Geometry check sheet. Reference: the model listing, model coordinates, mm. Face numbers are marked on the shaded views. Round coordinates to 2 decimals unless told otherwise and drop trailing zeros. Write each loop counter-clockwise with the first axis right and the second up, starting at its lowest first coordinate (ties: lowest second). Pieces come first, ordered by that corner, then holes. Notation, with made-up numbers: M -17.5,74 L 35.5,74 A21 ccw 35.5,92 Z; hole C 41,80.25 d11. An arc over 180 degrees is marked long. Use a Markdown table: item, result.
```python
from build123d import *

# Parameters (mm, degrees)
SKETCH1_W               = 22.5
SKETCH1_H               = 14
EXTRUDE1_DEPTH          = 7.2
SKETCH6_R               = 0.45
CUT_EXTRUDE1_DEPTH      = 0.1
CUT_EXTRUDE2_DEPTH      = 1
CUT_EXTRUDE2_DEPTH_BACK = 23.5
CUT_EXTRUDE3_DEPTH      = 1
CUT_EXTRUDE3_DEPTH_BACK = 15
LPATTERN1_COUNT         = 2
LPATTERN1_PITCH         = 7.5
LPATTERN2_COUNT         = 2
LPATTERN2_PITCH         = 7.5
BOSS_EXTRUDE4_START     = -1
SKETCH11_R              = 0.225
BOSS_EXTRUDE4_DEPTH     = 7.1
LPATTERN3_COUNT         = 6
LPATTERN3_PITCH         = 2.54
LPATTERN3_COUNT_DIR2    = 2
LPATTERN3_PITCH_DIR2    = 10.16


with BuildPart() as part:
    # Sketch1 → Extrude1 (new body)
    with BuildSketch(Plane(origin=(0, 0, 0), x_dir=(1, 0, 0), z_dir=(0, 1, 0))):
        Rectangle(SKETCH1_W, SKETCH1_H)
    extrude(amount=-EXTRUDE1_DEPTH)

    # Sketch6 → Cut-Extrude1 (cut)
    with BuildSketch(Plane(origin=(0, 0, 0), x_dir=(-1, 0, 0), z_dir=(0, 1, 0))):
        with Locations((-2.828914589, 5.1)):
            Circle(SKETCH6_R)
        Polygon((1.615140342, 0.645647316), (1.874984591, 3.615680666), (2.672057265, 4.346063205), (2.736318521, 4.281801948), (2.412096101, 0.575922722), (1.978755924, 0.212307139), align=None)
        Polygon((-2.08510989, 4.246446609), (-2.404999919, 0.590086851), (-2.118563171, 0.248724827), (-1.593244842, 0.689519243), (-1.335889658, 3.631102448), (-1.988382771, 4.343173729), align=None)
        Polygon((-2.751982586, -4.346963991), (-2.828914589, -4.255280001), (-2.499336567, -0.488185972), (-2.097293847, -0.150832074), (-1.707416581, -0.615469707), (-1.976986224, -3.696664829), align=None)
        Polygon((-2.591285684, -4.538475102), (-1.79792785, -3.872768836), (1.154576659, -3.872768836), (1.713170541, -4.538475102), (1.639848023, -4.6), (-2.539660165, -4.6), align=None)
        Polygon((1.560181456, -0.4), (1.954104558, -0.069459271), (1.560181456, 0.4), (-1.627135675, 0.4), (-2.021058776, 0.069459271), (-1.627135675, -0.4), align=None)
        Polygon((2.495112157, 4.523008313), (2.41812047, 4.6), (-1.7315565, 4.6), (-1.811437663, 4.520118836), (-1.151570324, 3.8), (1.706087039, 3.8), align=None)
        Polygon((1.982853172, -0.306417777), (2.30166085, -0.686357973), (1.984568022, -4.310745576), (1.904681652, -4.377778199), (1.244483112, -3.590984217), (1.496113015, -0.714841264), align=None)
    cut_extrude1 = extrude(amount=-CUT_EXTRUDE1_DEPTH, mode=Mode.SUBTRACT)

    # Sketch12 → Cut-Extrude2 (cut, two sides)
    with BuildSketch(Plane.ZY.offset(11.25)) as cut_extrude2_sk:
        Polygon((-20.043427491, -42.781711537), (-5.305, -7.2), (-4.890786438, -6.2), (4.890786438, -6.2), (5.305, -7.2), (20.043427491, -42.781711537), (20.043427491, -119.808445619), (-20.043427491, -119.808445619), align=None)
    extrude(amount=CUT_EXTRUDE2_DEPTH, mode=Mode.SUBTRACT)
    extrude(cut_extrude2_sk.sketch, amount=-CUT_EXTRUDE2_DEPTH_BACK, mode=Mode.SUBTRACT)

    # Sketch13 → Cut-Extrude3 (cut, two sides)
    with BuildSketch(Plane(origin=(0, 0, -7), x_dir=(-1, 0, 0), z_dir=(0, 0, -1))) as cut_extrude3_sk:
        Polygon((-32.290672921, -56.074755802), (-9.5, -7.2), (-9.033692342, -6.2), (9.033692342, -6.2), (9.5, -7.2), (32.290672921, -56.074755802), (32.290672921, -163.929408496), (-32.290672921, -163.929408496), align=None)
    extrude(amount=CUT_EXTRUDE3_DEPTH, mode=Mode.SUBTRACT)
    extrude(cut_extrude3_sk.sketch, amount=-CUT_EXTRUDE3_DEPTH_BACK, mode=Mode.SUBTRACT)

    # LPattern1: Cut-Extrude1 ×2
    with Locations(*[(i * LPATTERN1_PITCH, 0, 0) for i in range(1, LPATTERN1_COUNT)]):
        add(cut_extrude1, mode=Mode.SUBTRACT)

    # LPattern2: Cut-Extrude1 ×2
    with Locations(*[(-i * LPATTERN2_PITCH, 0, 0) for i in range(1, LPATTERN2_COUNT)]):
        add(cut_extrude1, mode=Mode.SUBTRACT)

    # Sketch11 → Boss-Extrude4 (add)
    with BuildSketch(Plane.XZ.offset(7.2).offset(BOSS_EXTRUDE4_START)):
        with Locations((6.35, 5.08)):
            Circle(SKETCH11_R)
    boss_extrude4 = extrude(amount=BOSS_EXTRUDE4_DEPTH)

    # LPattern3: Boss-Extrude4 6 × 2
    with Locations(*[(-i * LPATTERN3_PITCH, 0, -j * LPATTERN3_PITCH_DIR2) for i in range(LPATTERN3_COUNT) for j in range(LPATTERN3_COUNT_DIR2) if (i, j) != (0, 0)]):
        add(boss_extrude4)


solid = part.part
```
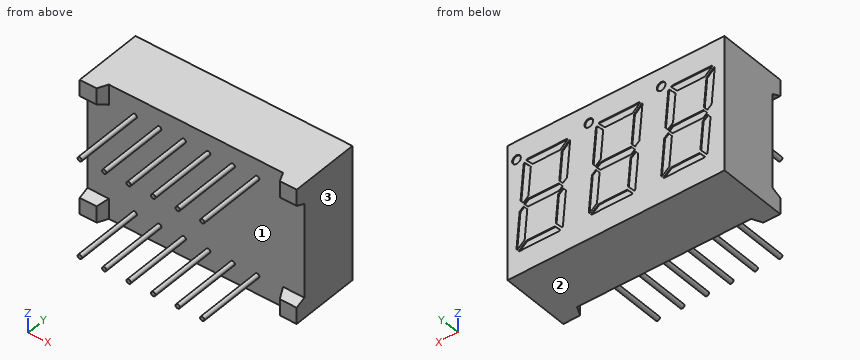
Item 1: Cross-section at C-C, the plane z = 2.25. Record the cut outline in (x, y).
Outcome:
| item | result |
|---|---|
| outline | M -11.25,-6.2 L 11.25,-6.2 L 11.25,0 L 9.76,0 L 9.76,-0.1 L 8.96,-0.1 L 8.96,0 L 5.74,0 L 5.74,-0.1 L 4.94,-0.1 L 4.94,0 L 2.26,0 L 2.26,-0.1 L 1.46,-0.1 L 1.46,0 L -1.76,0 L -1.76,-0.1 L -2.56,-0.1 L -2.56,0 L -5.24,0 L -5.24,-0.1 L -6.04,-0.1 L -6.04,0 L -9.26,0 L -9.26,-0.1 L -10.06,-0.1 L -10.06,0 L -11.25,0 Z |
Item 2: Cross-section at A-A, the plane y = -8.25. Count the separate pieces of the cut face and the enclosed holes in it, and give its area (3 significant figures).
Outcome:
| item | result |
|---|---|
| separate pieces | 12 |
| enclosed holes | 0 |
| area | 1.91 mm2 |
Item 3: Cross-section at B-B, the plane x = -3.25. Record the cut outline in (y, z).
Outcome:
| item | result |
|---|---|
| outline | M -6.2,-7 L 0,-7 L 0,7 L -6.2,7 Z |
Item 4: Mould release check, pull along X, two halves, no side actions. Record for the marked faces 1, 2 and 3: +X half, -X half, draft (parallel to the pull), parting line (faces both ways), or undercut.
Outcome:
| item | result |
|---|---|
| face 1 | undercut |
| face 2 | draft |
| face 3 | +X half |
Item 5: Material ranges on line 1 along Y through (x, z) = (-2.5, 2.25); line 2 along X through (y, z) = (-9.25, 5); line 3 along Y through (x, z) = (4.75, -3), recorded low to high. Write a range as from..to.
Outcome:
| item | result |
|---|---|
| line 1 | y = -6.2..-0.1 |
| line 2 | x = -6.56..-6.14, -4.02..-3.6, -1.48..-1.06, 1.06..1.48, 3.6..4.02, 6.14..6.56 |
| line 3 | y = -6.2..0 |
